```python
from build123d import *

# Parameters (mm, degrees)
F1_DEPTH     = 25.4
F3_DEPTH     = 101.6
F4_R         = 6.35
F6_D         = 12.7
F6_DEPTH     = 254
F6_TIP       = 3.8154649308
F7_T1_DEPTH  = 12.7
F7_T3_DEPTH  = 12.7
F7_T6_ANGLE  = 90
F7_T8_ANGLE  = 90
F7_T10_ANGLE = 90
F7_T12_ANGLE = 90


# Not quite as in the source:
# - a fillet or chamfer that OpenCascade refuses, or shapes differently, is made with other operations: its cross-section is extruded or revolved along the edge and cut away or added


with BuildPart() as f1:
    # F0 (on Front) → F1 (new body)
    with BuildSketch(Plane.XZ):
        Polygon((-12.7, -76.2), (0, -76.2), (12.7, -76.2), (12.7, 0), (-12.7, 0), align=None)
    extrude(amount=F1_DEPTH)

    # F2 (on face) → F3 (join)
    with BuildSketch(Plane.XZ.offset(25.4)):
        with BuildLine():
            ThreePointArc((5.715, -19.05), (4.0411152545, -15.0088847455), (0, -13.335))
            Line((0, -13.335), (0, -19.05))
            Line((0, -19.05), (0, -24.765))
            ThreePointArc((0, -24.765), (4.0411152545, -23.0911152545), (5.715, -19.05))
        make_face()
        with BuildLine():
            Line((0, -19.05), (0, -13.335))
            ThreePointArc((0, -13.335), (-5.715, -19.05), (0, -24.765))
            Line((0, -24.765), (0, -19.05))
        make_face()
    extrude(amount=F3_DEPTH)

    # F4
    f4_edges = [f1.edges().sort_by_distance(p)[0] for p in [
        (12.7, -25.4, -38.1),
        (12.7, 0, -38.1),
        (-12.7, -25.4, -38.1),
        (-12.7, 0, -38.1),
    ]]
    fillet(f4_edges, radius=F4_R)

    # F6
    with Locations(Plane.XZ.offset(25.4)):
        with Locations((0, -66.675)):
            Hole(F6_D / 2, depth=F6_DEPTH)
            with Locations((0, 0, -(F6_DEPTH + F6_TIP / 2))):  # 118° drill point
                Cone(0, F6_D / 2, F6_TIP, mode=Mode.SUBTRACT)

    # F7: fillet of radius 6.35 on 6 edges, made by hand

    # F7_s2 → F7_t1 (cut)
    with BuildSketch(Plane.XZ.offset(6.35)):
        with BuildLine():
            ThreePointArc((6.35, -76.2), (10.8401280605, -74.3401280605), (12.7, -69.85))
            Line((12.7, -69.85), (12.7, -76.2))
            Line((12.7, -76.2), (6.35, -76.2))
        make_face()
        with BuildLine():
            ThreePointArc((-6.35, -76.2), (-10.8401280605, -74.3401280605), (-12.7, -69.85))
            Line((-12.7, -69.85), (-12.7, -76.2))
            Line((-12.7, -76.2), (-6.35, -76.2))
        make_face()
    extrude(amount=F7_T1_DEPTH, mode=Mode.SUBTRACT)

    # F7_s4 → F7_t3 (cut)
    with BuildSketch(Plane.YZ.offset(-6.35)):
        with BuildLine():
            ThreePointArc((-19.05, -76.2), (-23.5401280605, -74.3401280605), (-25.4, -69.85))
            Line((-25.4, -69.85), (-25.4, -76.2))
            Line((-25.4, -76.2), (-19.05, -76.2))
        make_face()
        with BuildLine():
            ThreePointArc((-6.35, -76.2), (-1.8598719395, -74.3401280605), (0, -69.85))
            Line((0, -69.85), (0, -76.2))
            Line((0, -76.2), (-6.35, -76.2))
        make_face()
    extrude(amount=F7_T3_DEPTH, mode=Mode.SUBTRACT)

    # F7_s5 → F7_t6 (revolve, cut)
    with BuildSketch(Plane.XZ.offset(6.35)):
        with BuildLine():
            ThreePointArc((-6.35, -76.2), (-10.8401280605, -74.3401280605), (-12.7, -69.85))
            Line((-12.7, -69.85), (-12.7, -76.2))
            Line((-12.7, -76.2), (-6.35, -76.2))
        make_face()
    revolve(axis=Axis((-6.35, -6.35, -76.2), (0, 0, -1)), revolution_arc=F7_T6_ANGLE, mode=Mode.SUBTRACT)

    # F7_s7 → F7_t8 (revolve, cut)
    with BuildSketch(Plane.XZ.offset(19.05)):
        with BuildLine():
            ThreePointArc((-6.35, -76.2), (-10.8401280605, -74.3401280605), (-12.7, -69.85))
            Line((-12.7, -69.85), (-12.7, -76.2))
            Line((-12.7, -76.2), (-6.35, -76.2))
        make_face()
    revolve(axis=Axis((-6.35, -19.05, -76.2), (0, 0, 1)), revolution_arc=F7_T8_ANGLE, mode=Mode.SUBTRACT)

    # F7_s9 → F7_t10 (revolve, cut)
    with BuildSketch(Plane.XZ.offset(6.35)):
        with BuildLine():
            ThreePointArc((6.35, -76.2), (10.8401280605, -74.3401280605), (12.7, -69.85))
            Line((12.7, -69.85), (12.7, -76.2))
            Line((12.7, -76.2), (6.35, -76.2))
        make_face()
    revolve(axis=Axis((6.35, -6.35, -76.2), (0, 0, 1)), revolution_arc=F7_T10_ANGLE, mode=Mode.SUBTRACT)

    # F7_s11 → F7_t12 (revolve, cut)
    with BuildSketch(Plane.YZ.offset(6.35)):
        with BuildLine():
            ThreePointArc((-19.05, -76.2), (-23.5401280605, -74.3401280605), (-25.4, -69.85))
            Line((-25.4, -69.85), (-25.4, -76.2))
            Line((-25.4, -76.2), (-19.05, -76.2))
        make_face()
    revolve(axis=Axis((6.35, -19.05, -76.2), (0, 0, 1)), revolution_arc=F7_T12_ANGLE, mode=Mode.SUBTRACT)


solid = f1.part
```
Can you work these out from the model? Positions are in its coordinate system, mm. Give positions to 0.01 mm unless a question says otherwise; leave off trailing zeros. Write each loop counter-clockwise with the first axis right and the second up, starting at its lowest first coordinate (ties: lowest second). Pieces come first, ordered by that corner, then holes. Notation, with made-up numbers: (51.25, 35) - (59.25, 35) arc R15 cw to (59.25, 54) - close; hole circle Ø5 at (36, 48.25). An arc over 180 degrees is marked (long way). Write item = value, one per line. Start each with the question number.
1. Imagine slicing it at C-C (y = -21.5). Please give me the cut outline in (x, z) (3 decimals).
2. Thinking about a two-plate mould opening in Z: for faces 1 (the face through (1.377, -12.522, -72.874)), 2 (the face through (0, -13, 0)), 3 (the face through (-10.89, -1.91, -35.41)), which applies, released by +Z, released by -Z, zero draft, split by the parting line, or undercut?
3. Imagine slicing it at A-A (x = -2.25). Please give me the cut outline in (y, z).
4. Please list where these lines run through material, in increasing order: line 1 (Z direction, x = 0, y = -17.75) (3 decimals); line 2 (Z direction, x = -3.25, y = -16); line 3 (Y direction, x = -6, z = -63).
5. Imagine slicing it at D-D (y = -119). Please give me the cut outline in (x, z) (3 decimals), and give its area (3 significant figures).
6. Imagine slicing it at B-B (z = -48.5). Please give me the cut outline in (x, y), and give its area (3 significant figures).
7. For pin 1 (5 mm diameter, centred on x = 5, y = -64.5, fed in from -Z); pin 2 (2 mm diameter, centred on x = -3, z = -51, fed in from -Y); pin 3 (4 mm diameter, centred on x = -3, y = -26, fed in from -Z), each with a flat end and sliding along its axis, tell me the tip position at first contact or that it passes through.
Worked answers:
q1.outline = (-12.208, -69.85) arc R5.858 ccw to (-6.35, -75.708) - (6.35, -75.708) arc R5.858 ccw to (12.208, -69.85) - (12.208, 0) - (-12.208, 0) - close; hole circle Ø12.7 at (0, -66.675)
q2.face_1 = undercut
q2.face_2 = released by +Z
q2.face_3 = zero draft
q3.outline = (-127, -24.3) - (-25.4, -24.3) - (-25.4, -60.74) - (0, -60.74) - (0, 0) - (-25.4, 0) - (-25.4, -13.8) - (-127, -13.8) - close; (-24.77, -72.61) arc R6.35 ccw to (-19.05, -76.2) - (-6.35, -76.2) arc R6.35 ccw to (-0.63, -72.61) - close
q4.line_1 = -76.2 to -73.025, -60.325 to 0
q4.line_2 = -76.2 to -72.13, -61.22 to 0
q4.line_3 = -25.4 to 0
q5.outline = circle Ø11.43 at (0, -19.05)
q5.area = 103 mm2
q6.outline = (-12.7, -19.05) arc R6.35 ccw to (-6.35, -25.4) - (6.35, -25.4) arc R6.35 ccw to (12.7, -19.05) - (12.7, -6.35) arc R6.35 ccw to (6.35, 0) - (-6.35, 0) arc R6.35 ccw to (-12.7, -6.35) - close
q6.area = 611 mm2
q7.pin_1 = -24.19
q7.pin_2 = -25.4
q7.pin_3 = -73.83
